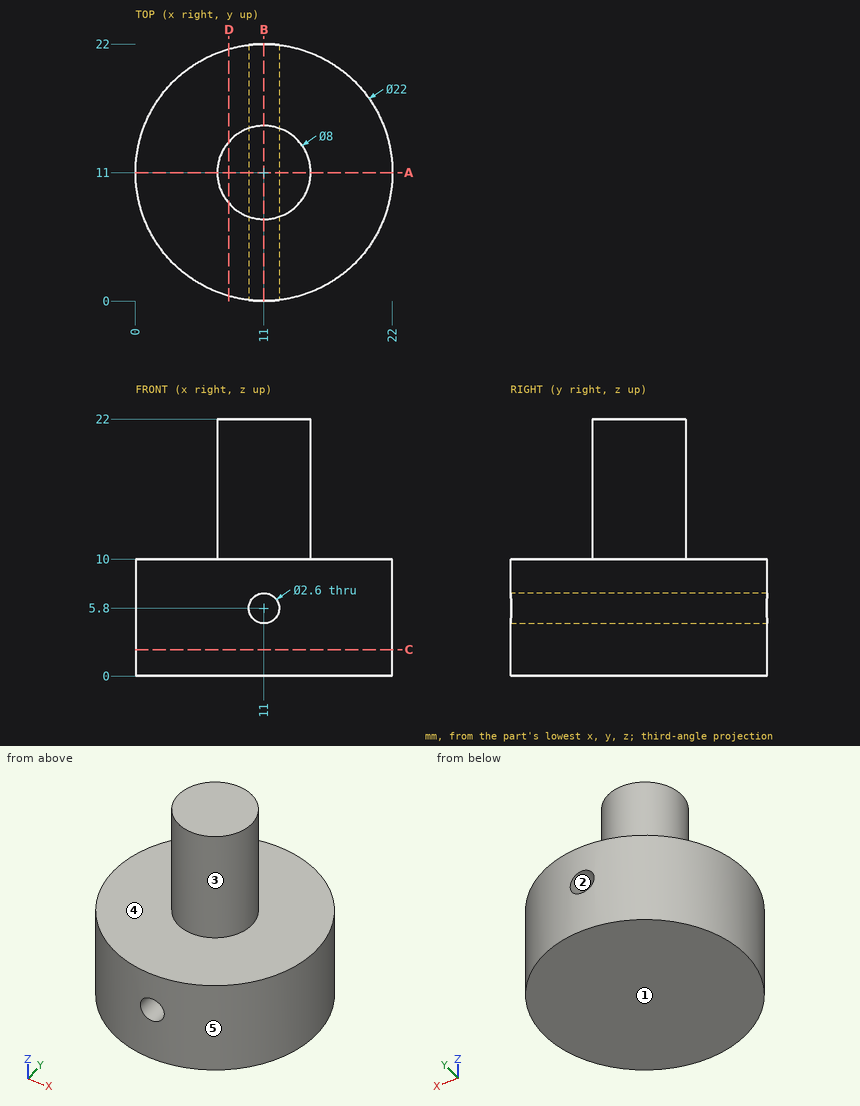
For this review, use the dimensioned drawing (mm, ordinates from the lowest corner) and the shaded views. A direction names the side the tool comes from. Give positions to 0.01 mm unless a question says otherwise; leave off trailing zeros. Order: outer loops, then holes, each group sorted by start corner. A loop starts at its lowest first (then second) coordinate and runs counter-clockwise, first axis right, second up.
1. Add section A-A, the plane y = 11. State the section outline as (x, z) points, then the cut area to 3 significant figures.
Solution:
outline: (0, 0) - (22, 0) - (22, 10) - (15, 10) - (15, 22) - (7, 22) - (7, 10) - (0, 10) - close; hole circle Ø2.6 at (11, 5.8)
area: 311 mm2
2. Tool access review of the marked faces 4 and 5: name each direction out of +Z, -Z, +X, -X, +Y, -Y from which nothing blocks a thin tool from reaching the whole face with its end or side.
Solution:
face 4: +Z
face 5: +Z, -Z
3. Add section D-D, the plane x = 8. State the section outline as (y, z) points.
Solution:
outline: (0.42, 0) - (21.58, 0) - (21.58, 10) - (13.65, 10) - (13.65, 22) - (8.35, 22) - (8.35, 10) - (0.42, 10) - close
4. Add section C-C, the plane z = 2.25. State the section outline as (x, y) points, then the cut area to 3 significant figures.
Solution:
outline: circle Ø22 at (11, 11)
area: 380 mm2
5. Add section B-B, the plane x = 11. State the section outline as (y, z) points.
Solution:
outline: (0, 0) - (22, 0) - (22, 4.5) - (0, 4.5) - close; (0, 7.1) - (22, 7.1) - (22, 10) - (15, 10) - (15, 22) - (7, 22) - (7, 10) - (0, 10) - close
6. Mouldability with a two-part tool opening along X and no side actions: class the marked faces 1, 2 and 3 as +X half, -X half, draft (parallel to the pull), parting line (faces both ways), or undercut.
Solution:
face 1: draft
face 2: undercut
face 3: parting line
7. To check wall thickness, follow L1, parallel to X at y = 10.75, z = 5.8; L2, parallel to Z at x = 19, y = 11.25; L3, parallel to X at y = 7, z = 5.8. State the ranges of each line that lie inside material, in increasing order.
Solution:
L1: x = 0 to 9.7, 12.3 to 22
L2: z = 0 to 10
L3: x = 0.75 to 9.7, 12.3 to 21.25
8. For pin 1 Ø4 at (x, z) = (11, 5.8) entering from +Y; pin 2 Ø2 at (y, z) = (3, 3.5) entering from -X; pin 3 Ø8 at (y, z) = (8.5, 16.5) entering from +X; pin 4 Ø6 at (x, y) = (19, 18) entering from +Z, all flat-tipped, find the tip position at first contact; note any pin that passes through.
Solution:
pin 1: stops at y = 22
pin 2: stops at x = 2.51
pin 3: stops at x = 15
pin 4: stops at z = 10
